CAD build for the part. Positions are in the model's coordinates, mm. A direction names the side the tool comes from. Give positions to 0.01 mm unless a question says otherwise; leave off trailing zeros. Write each loop counter-clockwise with the first axis right and the second up, starting at its lowest first coordinate (ties: lowest second). Pieces come first, ordered by that corner, then holes. Notation, with made-up numbers: (84, 84) -> (116, 84) arc R26 ccw to (116, 111) -> close; hole circle Ø3 at (77, 15). An arc over 180 degrees is marked (long way). Answer as a JSON object with one key per item and string values.
Autodesk Inventor part; units mm, degrees
ref_plane "YZ Plane" through (0, 0, 0) normal (1, 0, 0) x (0, 1, 0)
ref_plane "XZ Plane" through (0, 0, 0) normal (0, 1, 0) x (-1, 0, 0)
ref_plane "XY Plane" through (0, 0, 0) normal (0, 0, 1) x (1, 0, 0)
sketch "Эскиз1" plane through (0, 0, 0) normal (0, 1, 0) x (-1, 0, 0)
  line L0 (-18, -22.5) -> (18, -22.5)
  line L1 (18, -22.5) -> (18, 22.5)
  line L2 (18, 22.5) -> (-18, 22.5)
  line L3 (-18, 22.5) -> (-18, -22.5)
  line L4 (-18, -22.5) -> (18, 22.5) construction
  line L5 (18, -22.5) -> (-18, 22.5) construction
  circle A0 centre (15, -14) radius 1.5
  line L6 (0, -22.5) -> (0, 22.5) construction
  circle A1 centre (-15, -14) radius 1.5
  circle A2 centre (14.75, -18.5) radius 1.4
  circle A3 centre (-14.75, -18.5) radius 1.4
  point P0 (0, 0)
  dimension "d0" = 36
  dimension "d1" = 45
  dimension "d2" = 3
  dimension "d3" = 30
  dimension "d4" = 8.5
  dimension "d5" = 2.8
  dimension "d6" = 29.5
  dimension "d7" = 4
extrude "Выдавливание1" add sketch "Эскиз1" against normal blind 1.6
sketch "Эскиз2" plane through (0, 0, 0) normal (0, 1, 0) x (1, 0, 0)
  line L0 (18, 22.5) -> (-18, 22.5) construction
  line L1 (-18, 22.5) -> (-18, -22.5) construction
  line L2 (-18, -22.5) -> (18, -22.5) construction
  line L3 (18, -22.5) -> (18, 22.5) construction
  circle A0 centre (-15, 14) radius 1.5 construction
  circle A1 centre (15, 14) radius 1.5 construction
  circle A2 centre (-14.75, 18.5) radius 1.4 construction
  circle A3 centre (14.75, 18.5) radius 1.4 construction
  line L4 (-15, 14) -> (15, 14) construction
  line L5 (-18, 22.5) -> (18, 22.5) construction
  line L6 (0, 22.5) -> (0, 0) construction
  line L7 (-8.5, 22.6) -> (8.5, 22.6)
  line L8 (8.5, 22.6) -> (8.5, 5.6)
  line L9 (8.5, 5.6) -> (-8.5, 5.6)
  line L10 (-8.5, 5.6) -> (-8.5, 22.6)
  line L11 (-8.5, 5.6) -> (8.5, 22.6) construction
  line L12 (-8.5, 22.6) -> (8.5, 5.6) construction
  point P0 (0, 14.1)
  dimension "d10" = 17
  dimension "d11" = 17
  dimension "d12" = 0.1
extrude "Выдавливание2" add sketch "Эскиз2" along normal blind 9.6
sketch "Эскиз3" plane through (0, 9.6, 0) normal (0, 1, 0) x (1, 0, 0)
  line L0 (8.5, 22.6) -> (-8.5, 22.6)
  line L1 (-8.5, 22.6) -> (-8.5, 5.6)
  line L2 (-8.5, 5.6) -> (8.5, 5.6)
  line L3 (8.5, 5.6) -> (8.5, 22.6)
  line L4 (8.5, 22.6) -> (-8.5, 22.6) construction
  line L5 (8.5, 22.6) -> (-8.5, 5.6) construction
  line L6 (-8.5, 22.6) -> (-8.5, 5.6) construction
  line L7 (-8.5, 5.6) -> (8.5, 5.6) construction
  line L8 (-8.5, 22.6) -> (8.5, 5.6) construction
  circle A0 centre (0, 14.1) radius 7.5
  point P0 (0, 0)
  dimension "d15" = 15
extrude "Выдавливание3" add sketch "Эскиз3" along normal blind 6 contours A0
sketch "Эскиз4" plane through (0, 15.6, -14.1) normal (0, 1, 0) x (1, 0, 0)
  circle A0 centre (0, 0) radius 7.5
  circle A1 centre (0, 0) radius 7.7
  point P0 (0, -14.1)
  dimension "d18" = 15.4
extrude "Выдавливание4" add sketch "Эскиз4" along normal blind 3 contours A0 | A1
sketch "Эскиз5" plane through (0, 18.6, -14.1) normal (0, 1, 0) x (1, 0, 0)
  circle A0 centre (0, 0) radius 7.7
  circle A1 centre (0, 0) radius 6
  point P0 (0, -14.1)
  dimension "d21" = 12
extrude "Выдавливание5" add sketch "Эскиз5" along normal blind 3 contours A1
sketch "Эскиз6" plane through (0, 21.6, -14.1) normal (0, 1, 0) x (1, 0, 0)
  circle A0 centre (0, 0) radius 6
  circle A1 centre (0, 0) radius 7.5
  point P0 (0, -14.1)
  dimension "d24" = 15
extrude "Выдавливание6" add sketch "Эскиз6" along normal blind 3 contours A0 | A1
sketch "Эскиз7" plane through (0, 0, 0) normal (0, 1, 0) x (1, 0, 0)
  line L0 (-8.5, 5.6) -> (-8.5, 22.5) construction
  line L1 (-8.5, 22.5) -> (-18, 22.5) construction
  line L2 (-18, 22.5) -> (-18, -22.5) construction
  line L3 (-18, -22.5) -> (18, -22.5) construction
  line L4 (18, -22.5) -> (18, 22.5) construction
  line L5 (18, 22.5) -> (8.5, 22.5) construction
  line L6 (8.5, 22.5) -> (8.5, 5.6) construction
  line L7 (8.5, 5.6) -> (-8.5, 5.6) construction
  circle A0 centre (-15, 14) radius 1.5 construction
  circle A1 centre (15, 14) radius 1.5 construction
  circle A2 centre (-14.75, 18.5) radius 1.4 construction
  circle A3 centre (14.75, 18.5) radius 1.4 construction
  line L8 (5.5, -17) -> (13, -17)
  line L9 (13, -17) -> (13, -23)
  line L10 (13, -23) -> (5.5, -23)
  line L11 (5.5, -23) -> (5.5, -17)
  point P0 (0, 0)
  dimension "d27" = 7.5
  dimension "d28" = 6
  dimension "d29" = 5
  dimension "d32" = 0.5
extrude "Выдавливание7" add sketch "Эскиз7" along normal blind 3
properties part number "cam001"
1) Slice it at D-D (y = 5.75). List the corners of the cut face in (x, z), then the cut area to 3 significant figures.
Model answer:
{"outline": "(-8.5, -22.6) -> (8.5, -22.6) -> (8.5, -5.6) -> (-8.5, -5.6) -> close", "area": "289 mm2"}
2) Pin check, flat tips, straight feed: pin 1 (2 mm diameter, centred on x = -7, y = 7, fed in from +Z); pin 2 (2.5 mm diameter, centred on x = 15, z = -14, fed in from -Y); pin 3 (0.9 mm diameter, centred on x = 10.5, y = 1.5, fed in from -Z); pin 4 (6 mm diameter, centred on x = -10.5, y = 8.5, fed in from -Z). Stop position of each tip, or through.
Model answer:
{"pin 1": "stops at z = -5.6", "pin 2": "passes through", "pin 3": "stops at z = 17", "pin 4": "stops at z = -22.6"}
3) Slice it at C-C (x = 0). List the corners of the cut face in (y, z), then the cut area to 3 significant figures.
Model answer:
{"outline": "(-1.6, -22.5) -> (0, -22.5) -> (0, -22.6) -> (9.6, -22.6) -> (9.6, -21.6) -> (15.6, -21.6) -> (15.6, -21.8) -> (18.6, -21.8) -> (18.6, -20.1) -> (21.6, -20.1) -> (21.6, -21.6) -> (24.6, -21.6) -> (24.6, -6.6) -> (21.6, -6.6) -> (21.6, -8.1) -> (18.6, -8.1) -> (18.6, -6.4) -> (15.6, -6.4) -> (15.6, -6.6) -> (9.6, -6.6) -> (9.6, -5.6) -> (0, -5.6) -> (0, 22.5) -> (-1.6, 22.5) -> close", "area": "452 mm2"}
4) Slice it at B-B (x = 15). List the corners of the cut face in (y, z), then the cut area to 3 significant figures.
Model answer:
{"outline": "(-1.6, -22.5) -> (0, -22.5) -> (0, -19.88) -> (-1.6, -19.88) -> close; (-1.6, -17.12) -> (0, -17.12) -> (0, -15.5) -> (-1.6, -15.5) -> close; (-1.6, -12.5) -> (0, -12.5) -> (0, 22.5) -> (-1.6, 22.5) -> close", "area": "62.8 mm2"}
5) Slice it at A-A (z = -18.5). State how many separate pieces and enclosed holes the cut face has, then the cut area to 3 significant figures.
Model answer:
{"separate pieces": "3", "enclosed holes": "0", "area": "384 mm2"}
6) Mould opens along Y. For faces 1 (the flat face through (9, 3, 20)), 2 (the flat face through (2, 21.6, -20)), 3 (the cylindrical face through (15.86, -0.79, -19.35)) say: released by +Y, released by -Y, zero draft, split by the parting line, or undercut.
Model answer:
{"face 1": "released by +Y", "face 2": "undercut", "face 3": "zero draft"}
7) 3-axis set-ups, long thin cutter, end or side, ignore diameter. For faces 4 (the flat face through (5, 18.6, -10)), 5 (the cylindrical face through (-1.669, 17.079, -21.617)), 6 (the flat face through (0, -1, 22.5)): which of +Z, -Z, +X, -X, +Y, -Y reach the whole face in a straight line?
Model answer:
{"face 4": "none", "face 5": "+Y", "face 6": "+Z, +X, -X, -Y"}
8) Wall check: probe 1 along Y at (x, z) = (-6.5, -17); probe 2 along Z at (x, y) = (-15, -0.5); probe 3 along Z at (x, y) = (5.5, 6.5). Give the ranges that are in metal, low to high.
Model answer:
{"probe 1": "y = -1.6 to 18.6, 21.6 to 24.6", "probe 2": "z = -22.5 to -19.88, -17.12 to -15.5, -12.5 to 22.5", "probe 3": "z = -22.6 to -5.6"}
